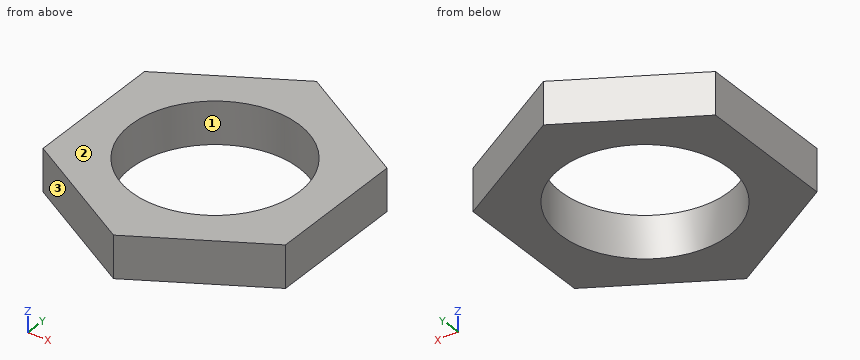
Autodesk Inventor part; units mm, degrees
ref_plane "YZ Plane" through (0, 0, 0) normal (1, 0, 0) x (0, 1, 0)
ref_plane "XZ Plane" through (0, 0, 0) normal (0, 1, 0) x (-1, 0, 0)
ref_plane "XY Plane" through (0, 0, 0) normal (0, 0, 1) x (1, 0, 0)
sketch "Эскиз1" plane through (0, 0, 0) normal (0, 0, 1) x (1, 0, 0)
  line L0 (0, -26.5581) -> (-23, -13.2791)
  line L1 (-23, -13.2791) -> (-23, 13.2791)
  line L2 (-23, 13.2791) -> (0, 26.5581)
  line L3 (0, 26.5581) -> (23, 13.2791)
  line L4 (23, 13.2791) -> (23, -13.2791)
  line L5 (23, -13.2791) -> (0, -26.5581)
  circle A0 centre (0, 0) radius 16
  dimension "d1" = 32
  dimension "d8" = 46
extrude "Выдавливание1" add sketch "Эскиз1" along normal blind 8
thread "Резьба1"
Here's how the part is built. I have some questions about the finished solid (model axes, mm). Face numbers are marked on the shaded views. Round coordinates to 2 decimals unless told otherwise and drop trailing zeros. Order: outer loops, then holes, each group sorted by start corner. A loop starts at its lowest first (then second) coordinate and runs counter-clockwise, first axis right, second up. Notation, with made-up numbers: M 51.5,46 L 64.5,46 A24 ccw 64.5,66 Z; hole C -36.75,88 d3. An arc over 180 degrees is marked long. Answer as CSV lines item,"result".
Item 1: Imagine slicing it at A-A on z = 3. List the corners of the cut face in (x, y) for me.
From the geometry:
outline,"M -23,-13.28 L 0,-26.56 L 23,-13.28 L 23,13.28 L 0,26.56 L -23,13.28 Z; hole C 0,0 d32"
Item 2: Imagine slicing it at B-B on y = 0. List the corners of the cut face in (x, z) for me.
From the geometry:
outline,"M -23,0 L -16,0 L -16,8 L -23,8 Z; M 16,0 L 23,0 L 23,8 L 16,8 Z"
Item 3: Imagine slicing it at C-C on x = 12. List the corners of the cut face in (y, z) for me, and give its area (3 significant figures).
From the geometry:
outline,"M -19.63,0 L -10.58,0 L -10.58,8 L -19.63,8 Z; M 10.58,0 L 19.63,0 L 19.63,8 L 10.58,8 Z"
area,"145 mm2"
Item 4: For pin 1 (2 mm diameter, centred on y = 15, z = 1, fed in from -X); pin 2 (1.5 mm diameter, centred on x = 7.5, z = 5.5, fed in from +Y), each with a flat end and sliding along its axis, tell me the tip position at first contact or that it passes through.
From the geometry:
pin 1,"x = -21.75"
pin 2,"y = 22.66"
Item 5: Imagine slicing it at D-D on x = 17. List the corners of the cut face in (y, z) for me.
From the geometry:
outline,"M -16.74,0 L 16.74,0 L 16.74,8 L -16.74,8 Z"
Item 6: Please list where these lines run through material, in increasing order: L1, parallel to Y at x = 0, z = 4.5; L2, parallel to X at y = 0.5, z = 3.25; L3, parallel to Y at x = 14, z = 3.75. Write a range as [from, to].
From the geometry:
L1,"[-26.56, -16], [16, 26.56]"
L2,"[-23, -15.99], [15.99, 23]"
L3,"[-18.48, -7.75], [7.75, 18.48]"
Item 7: We'd pull the mould along X, two halves only. Please class the marked faces 1, 2 and 3: +X half, -X half, draft (parallel to the pull), parting line (faces both ways), or undercut.
From the geometry:
face 1,"undercut"
face 2,"draft"
face 3,"-X half"
